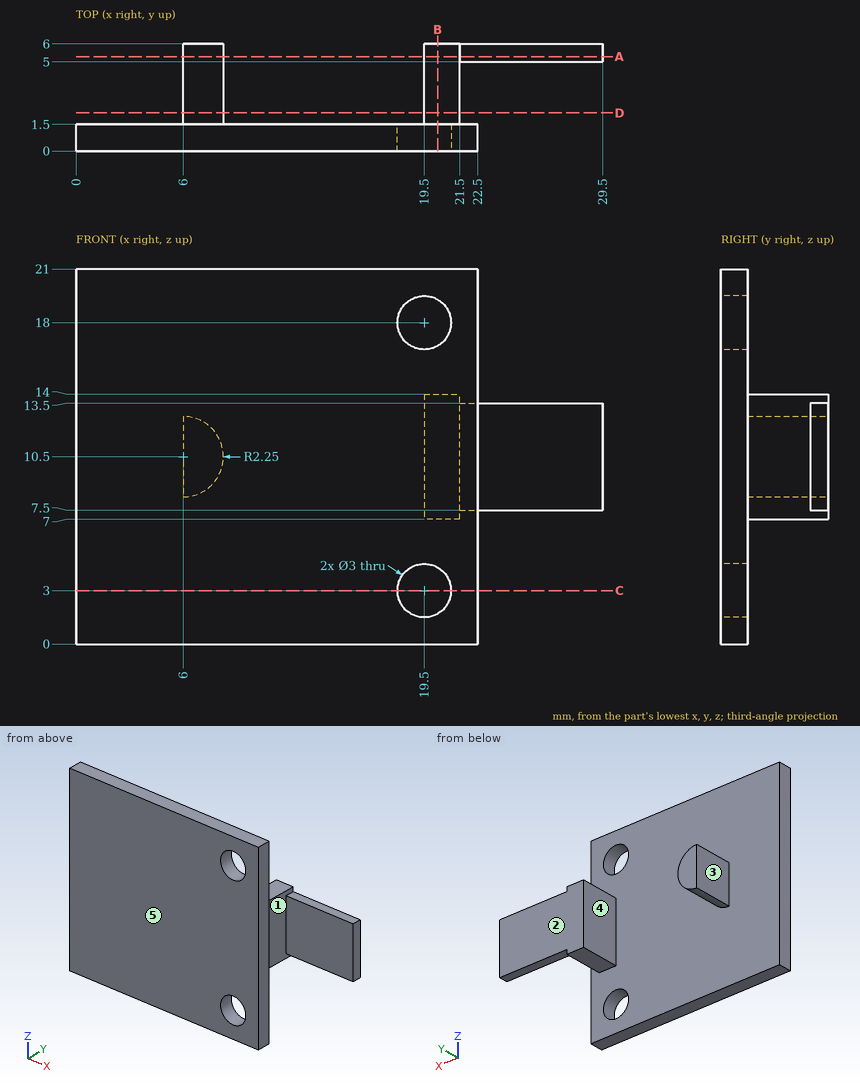
Geometry: see drawing. Coordinates: mm, zero at the bounding-box minimum. A direction names the side the tool comes from. Round coordinates to 2 decimals unless told otherwise and drop trailing zeros. Loops run counter-clockwise (first coordinate to the right, second up) from the corner with the lowest first, then second, coordinate; pieces in that order, holes last. Notation, with made-up numbers: (-11.5, 40.5) - (17.5, 40.5) arc R14 ccw to (17.5, 49.5) - close; hole circle Ø7 at (29, -31.75). An arc over 180 degrees is marked (long way). Write item = value, one per line. Start each with the question number.
(1) Section query D-D, the plane y = 2.15. Output: boundary loops of the cut face in (x, z), plus the area to 3 significant figures.
(2) Set-up query: the marked faces 4 and 5. Return all of +Z, -Z, +X, -X, +Y, -Y with unobstructed straight access to the full face (end or side cutting, diameter ignored); none if empty.
(3) Section query C-C, the plane z = 3. Output: boundary loops of the cut face in (x, y).
(4) Section query A-A, the plane y = 5.3. Output: boundary loops of the cut face in (x, z), plus the area to 3 significant figures.
(5) Pin query (flat end, axial travel): pin 1 (2 mm diameter, centred on y = 4, z = 9.5, fed in from -X); pin 2 (2 mm diameter, centred on y = 4.5, z = 15.5, fed in from +X); pin 3 (6.5 mm diameter, centred on x = 27, z = 10.5, fed in from -Y); pin 4 (1.6 mm diameter, centred on x = 20.5, y = 4.5, fed in from -Z). Return the tip coordinate at first contact, or that it passes through.
(6) Pull-direction query (Y, two-part tool) for the marked faces 1, 2 and 3; classes: +Y half, -Y half, draft (parallel to the pull), parting line (faces both ways), or undercut.
(7) Ray query, line 1 along Z through (x, y) = (19.5, 1.1); line 2 along X through (y, z) = (0.6, 14); line 3 along Y through (x, z) = (10, 3.5). Return the intervals inside material, ascending. Write a range as from..to.
(8) Section query B-B, the plane x = 20.25. Output: boundary loops of the cut face in (y, z), plus the area to 3 significant figures.
Conclusion:
q1.outline = (6, 8.25) arc R2.25 ccw to (6, 12.75) - close; (19.5, 7) - (21.5, 7) - (21.5, 14) - (19.5, 14) - close
q1.area = 22.0 mm2
q2.face_4 = +Z, -Z, +Y
q2.face_5 = +Z, -Z, +X, -X, -Y
q3.outline = (0, 0) - (18, 0) - (18, 1.5) - (0, 1.5) - close; (21, 0) - (22.5, 0) - (22.5, 1.5) - (21, 1.5) - close
q4.outline = (6, 8.25) arc R2.25 ccw to (6, 12.75) - close; (19.5, 7) - (21.5, 7) - (21.5, 7.5) - (29.5, 7.5) - (29.5, 13.5) - (21.5, 13.5) - (21.5, 14) - (19.5, 14) - close
q4.area = 70.0 mm2
q5.pin_1 = 6
q5.pin_2 = through
q5.pin_3 = 5
q5.pin_4 = 7
q6.face_1 = undercut
q6.face_2 = +Y half
q6.face_3 = draft
q7.line_1 = 0..1.5, 4.5..16.5, 19.5..21
q7.line_2 = 0..22.5
q7.line_3 = 0..1.5
q8.outline = (0, 0) - (1.5, 0) - (1.5, 1.7) - (0, 1.7) - close; (0, 4.3) - (1.5, 4.3) - (1.5, 7) - (6, 7) - (6, 14) - (1.5, 14) - (1.5, 16.7) - (0, 16.7) - close; (0, 19.3) - (1.5, 19.3) - (1.5, 21) - (0, 21) - close
q8.area = 55.2 mm2
